```python
from build123d import *

# Parameters (mm, degrees)
CROQUIS1_R              = 2.5
CROQUIS1_R_2            = 5
CROQUIS1_W              = 23
CROQUIS1_H              = 13
SALIENTE_EXTRUIR1_DEPTH = 2.5
CROQUIS2_W              = 4.5
CROQUIS2_H              = 13
SALIENTE_EXTRUIR2_DEPTH = 8


with BuildPart() as part:
    # Croquis1 → Saliente-Extruir1 (new body, symmetric)
    with BuildSketch(Plane.XY):
        with BuildLine():
            Line((30, 25), (-30, 25))
            ThreePointArc((-30, 25), (-35.857864376, 10.857864376), (-50, 5))
            Line((-50, 5), (-50, -75))
            Line((-50, -75), (0, -75))
            ThreePointArc((0, -75), (14.644660941, -39.644660941), (50, -25))
            Line((50, -25), (50, 5))
            ThreePointArc((50, 5), (35.857864376, 10.857864376), (30, 25))
        make_face()
        Circle(CROQUIS1_R, mode=Mode.SUBTRACT)
        with Locations((-28, 0)):
            Circle(CROQUIS1_R_2, mode=Mode.SUBTRACT)
        with Locations((28, 0)):
            Circle(CROQUIS1_R_2, mode=Mode.SUBTRACT)
        with Locations((-22.5, -56)):
            Rectangle(CROQUIS1_W, CROQUIS1_H, mode=Mode.SUBTRACT)
    extrude(amount=SALIENTE_EXTRUIR1_DEPTH, both=True)

    # Croquis2 → Saliente-Extruir2 (add)
    with BuildSketch(Plane.XY.offset(2.5)):
        with Locations((-36.25, -56)):
            Rectangle(CROQUIS2_W, CROQUIS2_H)
        with Locations((-8.75, -56)):
            Rectangle(CROQUIS2_W, CROQUIS2_H)
    extrude(amount=-SALIENTE_EXTRUIR2_DEPTH)


solid = part.part
```
CAD build for the part. Positions are in the model's coordinates, mm. A direction names the side the tool comes from. Give positions to 0.01 mm unless a question says otherwise; leave off trailing zeros. Write each loop counter-clockwise with the first axis right and the second up, starting at its lowest first coordinate (ties: lowest second). Pieces come first, ordered by that corner, then holes. Notation, with made-up numbers: (0, 26) -> (49, 26) arc R25 ccw to (49, 47) -> close; hole circle Ø10 at (82, 18.25). An arc over 180 degrees is marked (long way). Write each question's results on one line, items separated by ' | '.
1. Cut at B-B, the plane y = 0. Write the cut outline in (x, z).
Geometry check:
outline: (-50, -2.5) -> (-33, -2.5) -> (-33, 2.5) -> (-50, 2.5) -> close; (-23, -2.5) -> (-2.5, -2.5) -> (-2.5, 2.5) -> (-23, 2.5) -> close; (2.5, -2.5) -> (23, -2.5) -> (23, 2.5) -> (2.5, 2.5) -> close; (33, -2.5) -> (50, -2.5) -> (50, 2.5) -> (33, 2.5) -> close
2. Cut at D-D, the plane x = -9.5. Write the cut outline in (y, z), then the cut area to 3 significant figures.
Geometry check:
outline: (-75, -2.5) -> (-62.5, -2.5) -> (-62.5, -5.5) -> (-49.5, -5.5) -> (-49.5, -2.5) -> (25, -2.5) -> (25, 2.5) -> (-75, 2.5) -> close | area: 539 mm²
3. Drop flat-ended pins along their axis: P1, Ø2.5, axis at x = -35.5, z = -4.5, coming from the +Y side; P2, Ø3.5, axis at y = -56.5, z = -4.5, coming from the +X side; P3, Ø0.9, axis at y = -55.5, z = -3.5, coming from the -X side. Give the stop position or say it passes through.
Geometry check:
P1: y = -49.5 | P2: x = -6.5 | P3: x = -38.5
4. Cut at A-A, the plane x = -28. Write the cut outline in (y, z).
Geometry check:
outline: (-75, -2.5) -> (-62.5, -2.5) -> (-62.5, 2.5) -> (-75, 2.5) -> close; (-49.5, -2.5) -> (-5, -2.5) -> (-5, 2.5) -> (-49.5, 2.5) -> close; (5, -2.5) -> (25, -2.5) -> (25, 2.5) -> (5, 2.5) -> close
5. Which spindle directions (+Z, -Z, +X, -X, +Y, -Y) get a long thin tool onto all of the face, cutting with end or side? Do faces 1 (the flat face through (-36, -62.5, -4)), 2 (the flat face through (-6.5, -56, -4)), 3 (the flat face through (-38.5, -56, -4)), 4 (the flat face through (-23, -49.5, 0)). Say none if no direction does.
Geometry check:
face 1: -Z, +X, -X, -Y | face 2: -Z, +X, +Y, -Y | face 3: -Z, -X, +Y, -Y | face 4: +Z, -Z
6. Cut at C-C, the plane z = -4.25. Write the cut outline in (x, y), then the cut area to 3 significant figures.
Geometry check:
outline: (-38.5, -62.5) -> (-34, -62.5) -> (-34, -49.5) -> (-38.5, -49.5) -> close; (-11, -62.5) -> (-6.5, -62.5) -> (-6.5, -49.5) -> (-11, -49.5) -> close | area: 117 mm²
7. Two-plate mould, pull along X, no slides. Class faces 5 (the flat face through (-12, -24, 2.5)), 6 (the flat face through (-23, -62.5, 0)), 7 (the flat face through (50, -10, 0)): pulls with the +X half, pulls with the -X half, needs draft (parallel to the pull), parting line crosses it, or undercut.
Geometry check:
face 5: needs draft | face 6: undercut | face 7: pulls with the +X half
8. Wall check: probe 1 along Y at (x, z) = (-28, 0.45); probe 2 along X at (y, z) = (4, -1.25); probe 3 along Z at (x, y) = (40.5, 2.5). Give the ranges that are in metal, low to high. Write a range as [from, to].
Geometry check:
probe 1: [-75, -62.5], [-49.5, -5], [5, 25] | probe 2: [-50, -31], [-25, 25], [31, 50] | probe 3: [-2.5, 2.5]
